```python
from build123d import *

# Parameters (mm, degrees)
PAD015_DEPTH    = 25
SKETCH016_R     = 27
POCKET017_DEPTH = 25
SKETCH030_W     = 44.4306459714
SKETCH030_H     = 35
PAD022_DEPTH    = 25
SKETCH031_W     = 39.0651033717
SKETCH031_H     = 35
POCKET021_DEPTH = 36
SKETCH032_W     = 23
SKETCH032_H     = 22
POCKET022_DEPTH = 36
SKETCH041_R     = 2.5
POCKET024_DEPTH = 52.1614566717
SKETCH044_W     = 100
SKETCH044_H     = 4
PAD025_DEPTH    = 25
SKETCH066_R     = 2
POCKET030_DEPTH = 4


with BuildPart() as part:
    # Sketch015 → Pad015 (new body)
    with BuildSketch(Plane.XY):
        with BuildLine():
            ThreePointArc((22.2152888505, -18.6408406809), (0, 29), (-22.2152888505, -18.6408406809))
            Line((-22.2152888505, -18.6408406809), (22.2152888505, -18.6408406809))
        make_face()
    extrude(amount=PAD015_DEPTH)

    # Sketch016 → Pocket017 (cut)
    with BuildSketch(Plane.XY):
        Circle(SKETCH016_R)
    extrude(amount=POCKET017_DEPTH, mode=Mode.SUBTRACT)

    # Sketch030 → Pad022 (join)
    with BuildSketch(Plane.XY):
        with Locations((0, -36.1408)):
            Rectangle(SKETCH030_W, SKETCH030_H)
    extrude(amount=PAD022_DEPTH)

    # Sketch031 → Pocket021 (cut)
    with BuildSketch(Plane.XY):
        with Locations((0, -36.1408)):
            Rectangle(SKETCH031_W, SKETCH031_H)
    extrude(amount=POCKET021_DEPTH, mode=Mode.SUBTRACT)

    # Sketch032 → Pocket022 (cut)
    with BuildSketch(Plane.YZ):
        with Locations((-31.1408, 12.5)):
            Rectangle(SKETCH032_W, SKETCH032_H)
    extrude(amount=-POCKET022_DEPTH, mode=Mode.SUBTRACT)

    # Sketch041 → Pocket024 (cut, through all)
    with BuildSketch(Plane(origin=(-23.1604566717, 0, 0), x_dir=(0, -1, 0), z_dir=(-1, 0, 0))):
        with Locations((48.14, 8.085693)):
            Circle(SKETCH041_R)
    extrude(amount=-POCKET024_DEPTH, mode=Mode.SUBTRACT)

    # Sketch044 → Pad025 (join)
    with BuildSketch(Plane.XY):
        with Locations((-79, 2)):
            Rectangle(SKETCH044_W, SKETCH044_H)
        Polygon((-32, 4), (-27.017239, 10.090035), (-27.680943, -7.676853), (-32, 0), align=None)
    extrude(amount=PAD025_DEPTH)

    # Sketch066 (on Face20 of Pad025) → Pocket030 (cut)
    with BuildSketch(Plane.XZ):
        with Locations((-95.5, 10)):
            Circle(SKETCH066_R)
        with Locations((-85.5, 16)):
            Circle(SKETCH066_R)
        with Locations((-75.5, 10)):
            Circle(SKETCH066_R)
    extrude(amount=-POCKET030_DEPTH, mode=Mode.SUBTRACT)


solid = part.part
```
The listing builds one solid part. Answer for the finished solid, in the listing's coordinates (mm). A direction names the side the tool comes from. Round coordinates to 2 decimals unless told otherwise and drop trailing zeros. Order: outer loops, then holes, each group sorted by start corner. A loop starts at its lowest first (then second) coordinate and runs counter-clockwise, first axis right, second up. Notation, with made-up numbers: (72.25, -15.75) - (97.25, -15.75) arc R16 cw to (97.25, -9.75) - close; hole circle Ø11 at (61.5, -39.75). An arc over 180 degrees is marked (long way). Put each result on its own line as item: value. Start each with the question number.
(1) Given P1, Ø10, axis at y = 16, z = 12, coming from the -X side; P2, Ø8, axis at x = -10, z = 10, coming from the +Y side; P3, Ø5, axis at y = -27.5, z = 11, coming from the -X side, each flat-ended and moving along its own axis, determine where each tip first touches the part or whether it passes through.
(2) Find section A-A (z = 22). Give the vertices of the cut face in (x, y), plus the area to 3 significant figures.
(3) Find section D-D (y = -17). Give the vertices of the cut face in (x, z), plus the area to 3 significant figures.
(4) Find section B-B (y = -41). Give the vertices of the cut face in (x, z), plus the area to 3 significant figures.
(5) Straight lines are drawn through the part: probe 1 along X at (y, z) = (-43, 12); probe 2 along Z at (x, y) = (20, -48); probe 3 along Y at (x, z) = (-93, 18.5). For each, find the intervals that lie inside material, in ascending order. Write a range as from..to.
(6) Determine the mould class of faces 1 (the cylindrical face through (-73.592, 1.972, 10.601)), 2 (the flat face through (-27, -9, 0)), 3 (the cylindrical face through (-83.592, 1.972, 16.601)), 4 (the flat face through (-129, 2, 12)) for opening direction Z: released by +Z, released by -Z, zero draft, split by the parting line, or undercut.
(7) For faces 5 (the flat face through (-19.533, -44, 10)), 6 (the flat face through (-22.215, -44, 10)), 7 (the flat face through (22.215, -36, 12)), determine the directions among +Z, -Z, +X, -X, +Y, -Y from which every point of the face is accessible in a straight line to the end or side of a thin tool.
(8) Find section C-C (x = -85.5). Give the vertices of the cut face in (y, z).
Reply:
1. P1: x = -26.83
1. P2: y = 28.37
1. P3: x = 19.53
2. outline: (-129, 0) - (-32, 0) - (-28.2, -6.75) arc R29 ccw to (-22.22, -18.64) - (-22.22, -19.64) - (-19.53, -19.64) - (-19.53, -18.64) arc R27 cw (long way) to (19.53, -18.64) - (19.53, -53.64) - (22.22, -53.64) - (22.22, -18.64) arc R29 ccw (long way) to (-27.32, 9.71) - (-32, 4) - (-129, 4) - close; (-22.22, -53.64) - (-19.53, -53.64) - (-19.53, -42.64) - (-22.22, -42.64) - close
2. area: 802 mm^2
3. outline: (-23.49, 0) - (-20.98, 0) - (-20.98, 25) - (-23.49, 25) - close; (20.98, 0) - (23.49, 0) - (23.49, 25) - (20.98, 25) - close
3. area: 126 mm^2
4. outline: (-22.22, 0) - (-19.53, 0) - (-19.53, 1.5) - (-22.22, 1.5) - close; (-22.22, 23.5) - (-19.53, 23.5) - (-19.53, 25) - (-22.22, 25) - close; (19.53, 0) - (22.22, 0) - (22.22, 25) - (19.53, 25) - close
4. area: 75.1 mm^2
5. probe 1: -22.22..-19.53, 19.53..22.22
5. probe 2: 0..5.59, 10.58..25
5. probe 3: 0..4
6. face 1: undercut
6. face 2: released by -Z
6. face 3: undercut
6. face 4: zero draft
7. face 5: +Z, -Z, -Y
7. face 6: +Z, -Z, -X, -Y
7. face 7: +Z, -Z, +X, -Y
8. outline: (0, 0) - (4, 0) - (4, 14) - (0, 14) - close; (0, 18) - (4, 18) - (4, 25) - (0, 25) - close
